Autodesk Fusion 360 part; units mm, degrees
sketch "Sketch1" plane through (0, 0, 0) normal (0, 0, 1) x (1, 0, 0)
  line L0 (0, 0) -> (35, 0)
  line L1 (35, 30) -> (0, 30)
  line L2 (0, 30) -> (0, 0)
  circle A0 centre (35, 15) radius 2.25
  arc A1 (35, 0) -> (35, 30) centre (35, 15) ccw
  line L3 (15, 0) -> (15, 30)
  line L4 (15, 15) -> (0, 30) construction
  line L5 (7.5, 22.5) -> (7.5, 30) construction
  line L6 (7.5, 22.5) -> (0, 22.5) construction
  circle A2 centre (6.5, 23.5) radius 1
  circle A3 centre (8.5, 23.5) radius 1 construction
  circle A4 centre (8.5, 6.5) radius 1
  line L7 (15, 0) -> (0, 15) construction
  line L8 (7.5, 7.5) -> (7.5, 0) construction
  line L9 (7.5, 7.5) -> (15, 7.5) construction
  point P0 (40, 0)
  point P1 (15, 15)
  dimension "d1" = 30
  dimension "d7" = 35
  dimension "d8" = 35
  dimension "d9" = 4.5
  dimension "d14" = 2
  dimension "d36" = 2
extrude "Extrude1" add sketch "Sketch1" along normal blind 5 contours L0 L1 L2 L3 | L0 L1 A1 L3 | A0 | A2 | A4 makes body 1
hole "Hole1" at (8.5, 6.5, 0) at (6.5, 23.5, 0) direction (0, 0, 1) diameter 2 end through all counterbore diameter 2.3 counterbore depth 1 bodies 1 1
sketch "Sketch2" plane through (0, 0, 5) normal (0, 0, 1) x (-1, 0, 0)
  circle A0 centre (-8.5, -6.5) radius 1
  circle A1 centre (-6.5, -23.5) radius 1
  arc A2 (-35, 0) -> (-35, -30) centre (-35, -15) ccw
  line L0 (-35, -30) -> (0, -30)
  line L1 (0, -30) -> (0, 0)
  line L2 (0, 0) -> (-35, 0)
  circle A3 centre (-35, -15) radius 2.25
fillet "Fillet1" radius 2 3 edges at (17.5, 0, 0) (50, 15, 0) (17.5, 30, 0) on bodies 1
ref_plane "WorkPlane1" through (25, 15, 22.5) normal (0, 0, 1) x (1, 0, 0)
mirror "Mirror1" about plane through (25, 15, 22.5) normal (0, 0, 1) of bodies 1 makes body 2
extrude "Extrude2" cut sketch "Sketch2" against normal blind 4 contours A3 bodies 1
sketch "Sketch3" plane through (0, 0, 40) normal (0, 0, -1) x (1, 0, 0)
  circle A0 centre (8.5, -6.5) radius 1
  circle A1 centre (6.5, -23.5) radius 1
  arc A2 (35, -30) -> (35, 0) centre (35, -15) ccw
  line L0 (35, 0) -> (0, 0)
  line L1 (0, 0) -> (0, -30)
  line L2 (0, -30) -> (35, -30)
  line L3 (31.4, -14.9863) -> (24.4256, -25.1806)
  line L4 (35, -15) -> (24.8695, -28.0239) construction
  arc A3 (24.4256, -25.1806) -> (27.7346, -27.7544) centre (26.1588, -26.3663) ccw
  line L5 (35.8992, -18.4859) -> (27.7346, -27.7544)
  line L6 (31.4, -14.9863) -> (35.8992, -18.4859) construction
  arc A4 (35.8992, -18.4859) -> (31.4, -14.9863) centre (35, -15) ccw
  point P0 (35, -15)
  point P1 (35, -15)
  dimension "d30" = 4.2
  dimension "d31" = 5.7
  dimension "d32" = 16.5
  dimension "d33" = 7.2
extrude "Extrude3" cut sketch "Sketch3" against normal blind 2 contours L3 A3 L5 A4 bodies 2
hidden bodies 1
equation "d1 = breadth"
equation "breadth = 30 mm"
equation "length = 50 mm"
equation "d7 = length - d6"
equation "d8 = d7"
equation "d27 = ( 35 / 2 ) * 1 mm"
equation "d36 = d14"
Work out the finished part from the listing and answer in its coordinate system (mm). A direction names the side the tool comes from. Round coordinates to 2 decimals unless told otherwise and drop trailing zeros. Write each loop counter-clockwise with the first axis right and the second up, starting at its lowest first coordinate (ties: lowest second). Pieces come first, ordered by that corner, then holes.
1) Consider probe 1 along Y at (x, z) = (17, 43.1); probe 2 along X at (y, z) = (23.5, 41.3); probe 3 along X at (y, z) = (6.5, 44.45). Determine where each line is inside the solid, lowest interval first.
2) A cutting plane is placed at C-C on x = 32.5. Determine the outline of the cut face in (y, z).
3) A cutting plane is placed at B-B on z = 41.1. Determine the outline of the cut face in (x, y), and give its area (3 significant figures).
4) A cutting plane is placed at D-D on z = 44.5. Determine the outline of the cut face in (x, y), and give its area (3 significant figures).
5) Flat-ended cylindrical pins translate along their axes: P1, Ø3, axis at y = 5, z = 44, coming from the +X side; P2, Ø0.7, axis at x = 8, y = 6, coming from the +Z side; P3, Ø4.5, axis at x = 35, y = 15, coming from the -Z side. Find the tip coordinate at first contact, or state that the pin passes through.
6) Which of the six approach directions +Z, -Z, +X, -X, +Y, -Y give full straight-line access (tool end or side, diameter ignored) to faces 5 (the face through (7.8, 5.59, 44.49)), 6 (the face through (24, 15, 45)), 7 (the face through (31, 20, 42))?
7) A cutting plane is placed at A-A on x = 8.5. Determine the outline of the cut face in (y, z).
8) Determine the mould class of faces 1 (the face through (50, 15, 42)), 2 (the face through (7.277, 22.652, 44.493)), 3 (the face through (37.3, 12.23, 40.99)), 4 (the face through (25, 15, 40)) for opening direction Y: pulls with the +Y half, pulls with the -Y half, needs draft (parallel to the pull), parting line crosses it, or undercut.
Entries:
1. probe 1: y = 0 to 30
1. probe 2: x = 0 to 5.5, 7.5 to 25.58, 31.48 to 47.36
1. probe 3: x = 0 to 7.35, 9.65 to 46.6
2. outline: (0, 40) - (12.41, 40) - (12.41, 42) - (22.34, 42) - (22.34, 40) - (30, 40) - (30, 43) arc R2 ccw to (28, 45) - (2, 45) arc R2 ccw to (0, 43) - close
3. outline: (0, 0) - (35, 0) arc R15 ccw to (35, 30) - (0, 30) - close; hole circle Ø2 at (6.5, 23.5); hole circle Ø2 at (8.5, 6.5); hole (24.43, 25.18) - (31.4, 14.99) arc R3.6 ccw (long way) to (35.9, 18.49) - (27.73, 27.75) arc R2.1 ccw to start
3. area: 1,290 mm2
4. outline: (0, 0.68) - (35, 0.68) arc R14.32 ccw to (35, 29.32) - (0, 29.32) - close; hole circle Ø2.3 at (6.5, 23.5); hole circle Ø2.3 at (8.5, 6.5)
4. area: 1,320 mm2
5. P1: stops at x = 47.22
5. P2: stops at z = 44
5. P3: stops at z = 42
6. face 5: +Z
6. face 6: +Z, +X, -X, +Y, -Y
6. face 7: -Z
7. outline: (0, 40) - (5.5, 40) - (5.5, 44) - (5.35, 44) - (5.35, 45) - (2, 45) arc R2 ccw to (0, 43) - close; (7.5, 40) - (30, 40) - (30, 43) arc R2 ccw to (28, 45) - (7.65, 45) - (7.65, 44) - (7.5, 44) - close
8. face 1: parting line crosses it
8. face 2: undercut
8. face 3: undercut
8. face 4: needs draft
